Could you check a few things on this drawing? It's one solid part, dimensions in mm from its lowest x, y, z. Coordinates: 2 decimals unless noted, no trailing zeros. Loops run counter-clockwise (first coordinate to the right, second up) from the corner with the lowest first, then second, coordinate; pieces in that order, holes last. Notation, with made-up numbers: M 79.5,50.5 L 95.5,50.5 A19 ccw 95.5,57.5 Z; hole C 81,80.5 d4. An arc over 180 degrees is marked long. Use one line per item in the form item = value. Start each with the question number.
(1) Thinking about a two-plate mould opening in Y: for the marked faces 1, 2 and 3, which applies, +Y half, -Y half, draft (parallel to the pull), parting line (faces both ways), or undercut?
(2) Imagine slicing it at D-D, the plane z = 34. Please give me the cut outline in (x, y).
(3) Imagine slicing it at C-C, the plane x = 11.5. Please give me the cut outline in (y, z) (1 decimal), and give its area (3 significant figures).
(4) Will these pins go through, and if not, where does the flat tip stop? P1, Ø23.5, axis at x = 24.5, z = 24.5, coming from the -Y side; P2, Ø4.5, axis at x = 31.22, z = 31.22, coming from the +Y side; P3, Ø1, axis at y = 2.5, z = 27, coming from the +X side.
(5) Imagine slicing it at A-A, the plane z = 24.5. Please give me the cut outline in (x, y).
(6) Imagine slicing it at B-B, the plane y = 5.15. Please give me the cut outline in (x, z), and give its area (3 significant figures).
(7) Please list where these lines run through material, in increasing order: L1, parallel to Z at x = 24.5, y = 3.7; L2, parallel to Y at x = 42, z = 22; L3, parallel to Z at x = 38, y = 1 (1 decimal).
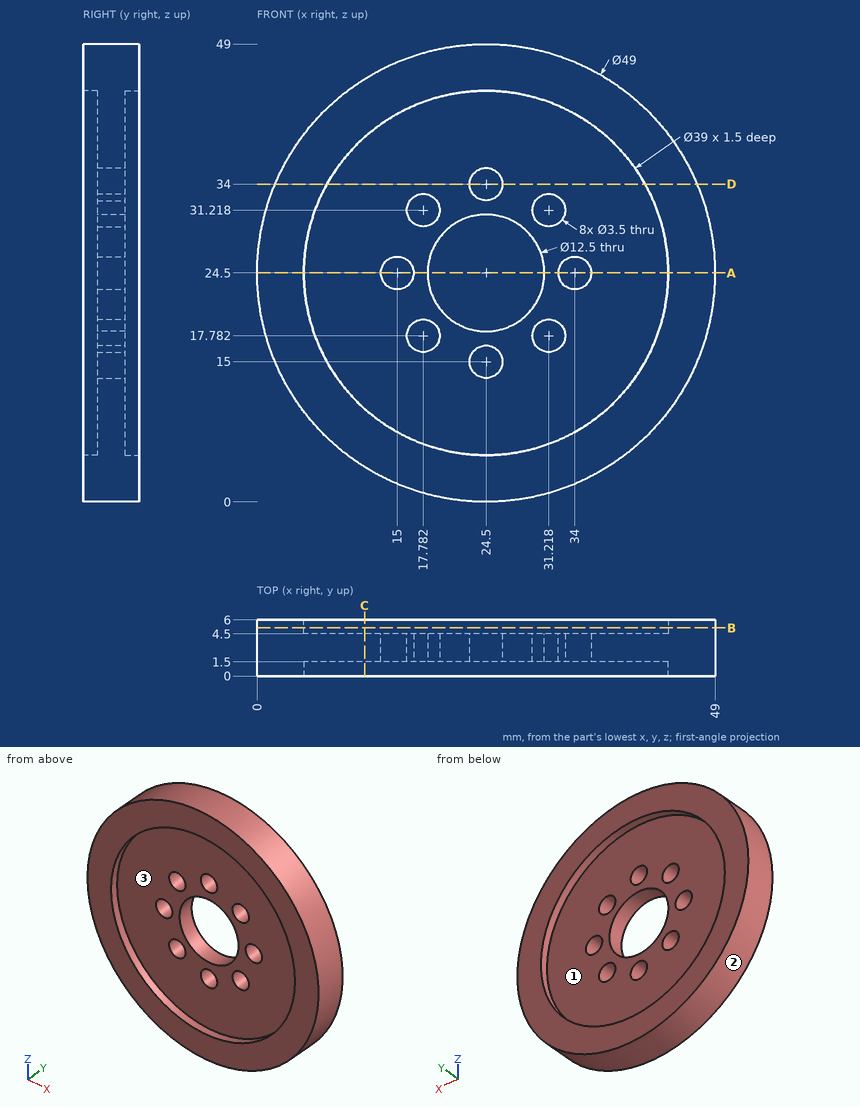
Answer:
q1.face_1 = +Y half
q1.face_2 = draft
q1.face_3 = -Y half
q2.outline = M 1.92,0 L 7.47,0 L 7.47,1.5 L 22.75,1.5 L 22.75,4.5 L 7.47,4.5 L 7.47,6 L 1.92,6 Z; M 26.25,1.5 L 41.53,1.5 L 41.53,0 L 47.08,0 L 47.08,6 L 41.53,6 L 41.53,4.5 L 26.25,4.5 Z
q3.outline = M 0,3.7 L 6,3.7 L 6,10 L 4.5,10 L 4.5,39 L 6,39 L 6,45.3 L 0,45.3 L 0,39 L 1.5,39 L 1.5,10 L 0,10 Z
q3.area = 162 mm²
q4.P1 = 1.5
q4.P2 = 4.5
q4.P3 = 48.92
q5.outline = M 0,0 L 5,0 L 5,1.5 L 13.25,1.5 L 13.25,4.5 L 5,4.5 L 5,6 L 0,6 Z; M 16.75,1.5 L 18.25,1.5 L 18.25,4.5 L 16.75,4.5 Z; M 30.75,1.5 L 32.25,1.5 L 32.25,4.5 L 30.75,4.5 Z; M 35.75,1.5 L 44,1.5 L 44,0 L 49,0 L 49,6 L 44,6 L 44,4.5 L 35.75,4.5 Z
q6.outline = C 24.5,24.5 d49; hole C 24.5,24.5 d39
q6.area = 691 mm²
q7.L1 = 0 to 13.25, 16.75 to 18.25, 30.75 to 32.25, 35.75 to 49
q7.L2 = 1.5 to 4.5
q7.L3 = 4.1 to 10.4, 38.6 to 44.9
